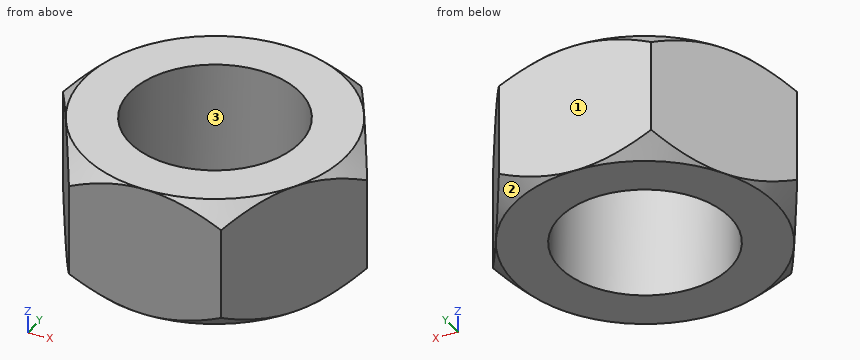
from build123d import *

# Parameters (mm, degrees)
CROQUIS1_R              = 7.14375
SALIENTE_EXTRUIR1_DEPTH = 11
CROQUIS2_R              = 31.223063066
CROQUIS2_R_2            = 11
CORTAR_EXTRUIR1_DEPTH   = 10
CORTAR_EXTRUIR1_DRAFT   = -46
CROQUIS4_R              = 40.862675885
CROQUIS4_R_2            = 11
CORTAR_EXTRUIR3_DEPTH   = 10
CORTAR_EXTRUIR3_DRAFT   = -46


with BuildPart() as part:
    # Croquis1 → Saliente-Extruir1 (new body)
    with BuildSketch(Plane.XY):
        Polygon((12.701705922, 0), (6.350852961, 11), (-6.350852961, 11), (-12.701705922, 0), (-6.350852961, -11), (6.350852961, -11), align=None)
        Circle(CROQUIS1_R, mode=Mode.SUBTRACT)
    extrude(amount=SALIENTE_EXTRUIR1_DEPTH)


with BuildPart() as cortar_extruir1_tool:
    # Croquis2 → Cortar-Extruir1 (with draft: the straight prism first)
    with BuildSketch(Plane.XY.offset(11)):
        Circle(CROQUIS2_R)
        Circle(CROQUIS2_R_2, mode=Mode.SUBTRACT)
    extrude(amount=-CORTAR_EXTRUIR1_DEPTH)
    # Cortar-Extruir1: the draft: its side faces are tilted about the plane it starts from
    cortar_extruir1_sides = [cortar_extruir1_tool.faces().sort_by_distance(p)[0] for p in [
        (-31.223063066, 0, 6),
        (-11, 0, 6),
    ]]
    draft(cortar_extruir1_sides, Plane.XY.offset(11), CORTAR_EXTRUIR1_DRAFT)


with BuildPart() as part_1:
    add(part.part)

    # Cortar-Extruir1: cut by cortar_extruir1_tool
    add(cortar_extruir1_tool.part, mode=Mode.SUBTRACT)


with BuildPart() as cortar_extruir3_tool:
    # Croquis4 → Cortar-Extruir3 (with draft: the straight prism first)
    with BuildSketch(Plane(origin=(0, 0, 0), x_dir=(-1, 0, 0), z_dir=(0, 0, -1))):
        Circle(CROQUIS4_R)
        Circle(CROQUIS4_R_2, mode=Mode.SUBTRACT)
    extrude(amount=-CORTAR_EXTRUIR3_DEPTH)
    # Cortar-Extruir3: the draft: its side faces are tilted about the plane it starts from
    cortar_extruir3_sides = [cortar_extruir3_tool.faces().sort_by_distance(p)[0] for p in [
        (40.862675885, 0, 5),
        (11, 0, 5),
    ]]
    draft(cortar_extruir3_sides, Plane(origin=(0, 0, 0), x_dir=(-1, 0, 0), z_dir=(0, 0, -1)), CORTAR_EXTRUIR3_DRAFT)


with BuildPart() as part_2:
    add(part_1.part)

    # Cortar-Extruir3: cut by cortar_extruir3_tool
    add(cortar_extruir3_tool.part, mode=Mode.SUBTRACT)


solid = part_2.part
Verification items for the finished model (mm, model axes). Face numbers are marked on the shaded views. Coordinates: 2 decimals unless noted, no trailing zeros. Loops run counter-clockwise (first coordinate to the right, second up) from the corner with the lowest first, then second, coordinate; pieces in that order, holes last. Notation, with made-up numbers: (-16, 74) -> (22, 74) arc R6 cw to (22, 81) -> close; hole circle Ø7 at (-7.75, 23). An arc over 180 degrees is marked (long way). Answer as a JSON object with one key per item and string values. Group by question number.
Item 1: Sectioned sample at A-A on z = 5.5. Record the boundary of the cut face in (x, y), plus the area to 3 significant figures.
Item 2: Depth check by flat-ended pin: pin 1 (3 mm diameter, centred on y = 0, z = 5.5, fed in from +X); pin 2 (5 mm diameter, centred on y = 6, z = 8.5, fed in from -X); pin 3 (3 mm diameter, centred on y = 2.5, z = 3, fed in from -X). Enter the tip coordinate at first touch or a pass-through.
Item 3: Scan lines: probe 1 along Y at (x, z) = (0, 5.75); probe 2 along Y at (x, z) = (6.25, 7); probe 3 along X at (y, z) = (0.5, 0.75). Record each from-to range of solid material in increasing order.
Item 4: Mould release check, pull along X, two halves, no side actions. Record for the marked faces 1, 2 and 3: +X half, -X half, draft (parallel to the pull), parting line (faces both ways), or undercut.
Item 5: Sectioned sample at B-B on z = 1. Record the boundary of the cut face in (x, y), plus the area to 3 significant figures.
Evaluation:
{
 "1": {"outline": "(-12.7, 0) -> (-6.35, -11) -> (6.35, -11) -> (12.7, 0) -> (6.35, 11) -> (-6.35, 11) -> close; hole circle Ø14.29 at (0, 0)", "area": "259 mm²"},
 "2": {"pin 1": "stops at x = 12.7", "pin 2": "stops at x = -10.68", "pin 3": "stops at x = -12.12"},
 "3": {"probe 1": "y = -11 to -7.14, 7.14 to 11", "probe 2": "y = -11 to -3.46, 3.46 to 11", "probe 3": "x = -11.77 to -7.13, 7.13 to 11.77"},
 "4": {"face 1": "draft", "face 2": "+X half", "face 3": "undercut"},
 "5": {"outline": "(-11.97, -1.27) -> (-7.08, -9.73) arc R12.04 ccw to (-4.88, -11) -> (4.88, -11) arc R12.04 ccw to (7.08, -9.73) -> (11.97, -1.27) arc R12.04 ccw to (11.97, 1.27) -> (7.08, 9.73) arc R12.04 ccw to (4.88, 11) -> (-4.88, 11) arc R12.04 ccw to (-7.08, 9.73) -> (-11.97, 1.27) arc R12.04 ccw to start; hole circle Ø14.29 at (0, 0)", "area": "254 mm²"}
}
